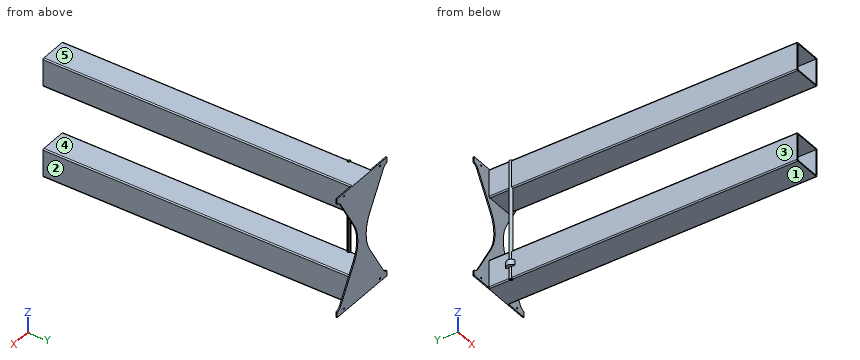
from build123d import *
from build123d.topology import SkipClean

# Parameters (mm, degrees)
SKETCH1_R           = 1.5875
BOSS_EXTRUDE1_DEPTH = 2.54
SKETCH2_W           = 63.5
SKETCH2_H           = 63.5
BOSS_EXTRUDE2_DEPTH = 685.8
SHELL1_START        = -688.34
SHELL1_OUTLINE_W    = 58.42
SHELL1_OUTLINE_H    = 58.42
SHELL1_DEPTH        = 685.8
FILLET1_R           = 2.54
FILLET2_R           = 2.54
CUT_EXTRUDE1_DEPTH  = 267.97
BOSS_EXTRUDE4_DEPTH = 27.94
BOSS_EXTRUDE5_DEPTH = 10.16
BOSS_EXTRUDE6_START = -0.762
BOSS_EXTRUDE6_DEPTH = 0.762
BOSS_EXTRUDE7_DEPTH = 0.762
BOSS_EXTRUDE8_DEPTH = 229.108
SKETCH12_W          = 2.54
SKETCH12_H          = 18.920978
CUT_EXTRUDE2_DEPTH  = 10.16


# Read off the part's stored shape, not the designer's step: Shell1
with BuildPart() as part:
    # Sketch1 → Boss-Extrude1 (new body)
    with BuildSketch(Plane(origin=(0, 0, 0), x_dir=(1, 0, 0), z_dir=(0, 1, 0))):
        with BuildLine():
            Line((-79.375, -133.985), (79.375, -133.985))
            Line((79.375, -133.985), (79.375, -123.618732))
            ThreePointArc((79.375, -123.618732), (78.770533, -121.973949), (77.244833, -121.112014))
            ThreePointArc((77.244833, -121.112014), (71.931312, -118.986411), (68.016546, -114.811929))
            Line((68.016546, -114.811929), (24.542449, -41.427653))
            ThreePointArc((24.542449, -41.427653), (13.192327, 0), (24.542449, 41.427653))
            Line((24.542449, 41.427653), (68.016546, 114.811929))
            ThreePointArc((68.016546, 114.811929), (71.931312, 118.986411), (77.244833, 121.112014))
            ThreePointArc((77.244833, 121.112014), (78.770533, 121.973949), (79.375, 123.618732))
            Line((79.375, 123.618732), (79.375, 133.985))
            Line((79.375, 133.985), (-79.375, 133.985))
            Line((-79.375, 133.985), (-79.375, 123.618732))
            ThreePointArc((-79.375, 123.618732), (-78.770533, 121.973949), (-77.244833, 121.112014))
            ThreePointArc((-77.244833, 121.112014), (-71.931312, 118.986411), (-68.016546, 114.811929))
            Line((-68.016546, 114.811929), (-24.542449, 41.427653))
            ThreePointArc((-24.542449, 41.427653), (-13.192327, 0), (-24.542449, -41.427653))
            Line((-24.542449, -41.427653), (-68.016546, -114.811929))
            ThreePointArc((-68.016546, -114.811929), (-71.931312, -118.986411), (-77.244833, -121.112014))
            ThreePointArc((-77.244833, -121.112014), (-78.770533, -121.973949), (-79.375, -123.618732))
            Line((-79.375, -123.618732), (-79.375, -133.985))
        make_face()
        with Locations(Location((-57.15, 127, 0), (0, 0, 270))):
            Circle(SKETCH1_R, mode=Mode.SUBTRACT)
        with Locations(Location((57.15, 127, 0), (0, 0, 270))):
            Circle(SKETCH1_R, mode=Mode.SUBTRACT)
        with Locations(Location((57.15, -127, 0), (0, 0, 90))):
            Circle(SKETCH1_R, mode=Mode.SUBTRACT)
        with Locations(Location((-57.15, -127, 0), (0, 0, 90))):
            Circle(SKETCH1_R, mode=Mode.SUBTRACT)
    extrude(amount=-BOSS_EXTRUDE1_DEPTH)

    # Sketch2 → Boss-Extrude2 (add)
    with BuildSketch(Plane.XZ.offset(2.54)):
        with Locations((0, -102.235)):
            Rectangle(SKETCH2_W, SKETCH2_H)
        with Locations((0, 102.235)):
            Rectangle(SKETCH2_W, SKETCH2_H)
    extrude(amount=BOSS_EXTRUDE2_DEPTH)

    # Shell1 outline → Shell1 (cut)
    with BuildSketch(Plane(origin=(0, 0, 0), x_dir=(1, 0, 0), z_dir=(0, 1, 0)).offset(SHELL1_START)):
        with Locations((0, 102.235)):
            Rectangle(SHELL1_OUTLINE_W, SHELL1_OUTLINE_H)
        with Locations((0, -102.235)):
            Rectangle(SHELL1_OUTLINE_W, SHELL1_OUTLINE_H)
    extrude(amount=SHELL1_DEPTH, mode=Mode.SUBTRACT)

    # Fillet1
    fillet1_edges = [part.edges().sort_by_distance(p)[0] for p in [
        (31.75, -345.44, 70.485),
        (31.75, -345.44, 133.985),
        (-31.75, -345.44, 133.985),
        (-31.75, -345.44, 70.485),
    ]]
    fillet(fillet1_edges, radius=FILLET1_R)

    # Fillet2
    fillet2_edges = [part.edges().sort_by_distance(p)[0] for p in [
        (-31.75, -345.44, -70.485),
        (-31.75, -345.44, -133.985),
        (31.75, -345.44, -133.985),
        (31.75, -345.44, -70.485),
    ]]
    fillet(fillet2_edges, radius=FILLET2_R)

    # Sketch4 → Cut-Extrude1 (cut)
    with BuildSketch(Plane(origin=(0, 0, -133.985), x_dir=(-1, 0, 0), z_dir=(0, 0, -1))):
        with BuildLine():
            ThreePointArc((29.21, -53.213), (31.455064, -52.283064), (32.385, -50.038))
            ThreePointArc((32.385, -50.038), (31.455064, -47.792936), (29.21, -46.863))
            Line((29.21, -46.863), (29.21, -53.213))
        make_face()
        with BuildLine():
            Line((29.21, -53.213), (29.21, -46.863))
            ThreePointArc((29.21, -46.863), (26.035, -50.038), (29.21, -53.213))
        make_face()
    extrude(amount=-CUT_EXTRUDE1_DEPTH, mode=Mode.SUBTRACT)

    # Sketch6 → Boss-Extrude4 (add)
    with BuildSketch(Plane(origin=(0, 0, -133.985), x_dir=(-1, 0, 0), z_dir=(0, 0, -1))):
        with BuildLine():
            Line((29.21, -46.863), (29.21, -46.228))
            ThreePointArc((29.21, -46.228), (33.02, -50.038), (29.21, -53.848))
            Line((29.21, -53.848), (29.21, -53.213))
            ThreePointArc((29.21, -53.213), (32.385, -50.038), (29.21, -46.863))
        make_face()
    extrude(amount=-BOSS_EXTRUDE4_DEPTH)

    # Sketch7 → Boss-Extrude5 (add)
    with BuildSketch(Plane.XY.offset(-106.045)):
        with BuildLine():
            ThreePointArc((-31.75, -40.069511), (-39.497, -50.038), (-31.75, -60.006489))
            Line((-31.75, -60.006489), (-31.75, -59.218089))
            ThreePointArc((-31.75, -59.218089), (-38.735, -50.038), (-31.75, -40.857911))
            Line((-31.75, -40.857911), (-31.75, -40.069511))
        make_face()
    extrude(amount=BOSS_EXTRUDE5_DEPTH)

    # Sketch7<2> → Boss-Extrude6 (add)
    with BuildSketch(Plane.XY.offset(-106.045).offset(BOSS_EXTRUDE6_START)):
        with BuildLine():
            ThreePointArc((-31.75, -40.069511), (-39.497, -50.038), (-31.75, -60.006489))
            Line((-31.75, -60.006489), (-31.75, -59.218089))
            ThreePointArc((-31.75, -59.218089), (-38.735, -50.038), (-31.75, -40.857911))
            Line((-31.75, -40.857911), (-31.75, -40.069511))
        make_face()
        with BuildLine():
            ThreePointArc((-31.75, -40.857911), (-38.735, -50.038), (-31.75, -59.218089))
            Line((-31.75, -59.218089), (-31.75, -52.877806))
            ThreePointArc((-31.75, -52.877806), (-33.02, -50.038), (-31.75, -47.198194))
            Line((-31.75, -47.198194), (-31.75, -40.857911))
        make_face()
    extrude(amount=BOSS_EXTRUDE6_DEPTH)

    # Sketch8 → Boss-Extrude7 (add)
    with SkipClean():  # the faces are left unmerged after this step: merging them gives an invalid solid
        with BuildSketch(Plane.XY.offset(-95.885)):
            with BuildLine():
                Line((-31.75, -40.069511), (-31.75, -48.133))
                ThreePointArc((-31.75, -48.133), (-32.385, -50.038), (-31.75, -51.943))
                Line((-31.75, -51.943), (-31.75, -60.006489))
                ThreePointArc((-31.75, -60.006489), (-39.497, -50.038), (-31.75, -40.069511))
            make_face()
        extrude(amount=BOSS_EXTRUDE7_DEPTH)

    # Sketch9 → Boss-Extrude8 (add)
    with SkipClean():  # the faces are left unmerged after this step: merging them gives an invalid solid
        with BuildSketch(Plane.XY.offset(-95.123)):
            with BuildLine():
                Line((-29.21, -46.228), (-29.21, -46.863))
                ThreePointArc((-29.21, -46.863), (-30.629903, -47.198194), (-31.75, -48.133))
                ThreePointArc((-31.75, -48.133), (-32.385, -50.038), (-31.75, -51.943))
                ThreePointArc((-31.75, -51.943), (-30.629903, -52.877806), (-29.21, -53.213))
                Line((-29.21, -53.213), (-29.21, -53.848))
                ThreePointArc((-29.21, -53.848), (-33.02, -50.038), (-29.21, -46.228))
            make_face()
        extrude(amount=BOSS_EXTRUDE8_DEPTH)

    # Sketch12 → Cut-Extrude2 (cut)
    with BuildSketch(Plane(origin=(0, 0, -95.885), x_dir=(-1, 0, 0), z_dir=(0, 0, -1))):
        with Locations((30.48, -50.038)):
            Rectangle(SKETCH12_W, SKETCH12_H)
    extrude(amount=CUT_EXTRUDE2_DEPTH, mode=Mode.SUBTRACT)


solid = part.part
Check sheet for the modelled part. Datum: model origin and axes. Units: mm. Face numbers are marked on the shaded views. A direction names the side the tool comes from. Round coordinates to 2 decimals unless told otherwise and drop trailing zeros. Write each loop counter-clockwise with the first axis right and the second up, starting at its lowest first coordinate (ties: lowest second). Pieces come first, ordered by that corner, then holes. Notation, with made-up numbers: (77.5, -13) -> (84.5, -13) arc R19 ccw to (84.5, 6) -> close; hole circle Ø9 at (24.5, 66.5). An arc over 180 degrees is marked (long way). Answer as CSV lines item,"result". Start each with the question number.
1) Section check B-B on z = -15.5. Enter the section's corners in (x, y) (3 decimals), and give its area (3 significant figures).
2) Section check A-A on y = -162. Enter the section's corners in (x, z) (3 decimals).
3) Section check C-C on x = -49. Enter the section's corners in (y, z) (3 decimals).
4) Section check D-D on x = -3. Enter the section's corners in (y, z) (3 decimals).
5) Material ranges on line 1 (X direction, y = -1, z = 127) (1 decimal); line 2 (Z direction, x = -4.5, y = -624.5) (3 decimals); line 3 (X direction, y = -635, z = 77), recorded low to high. Write a range as from..to.
6) Tool access check on the marked faces 1 and 2. Record the directions out of +Z, -Z, +X, -X, +Y, -Y that give a thin tool (end or side, any length) a straight path to the whole face; none if there is none.
7) Go/stop test with flat-tipped pins: P1, Ø10, axis at y = -291.5, z = -96.5, coming from the +X side; P2, Ø2.5, axis at x = -37.5, y = -49, coming from the +Z side; P3, Ø8.5, axis at x = -34, y = -49, coming from the -Z side (3 decimals); P4, Ø12, axis at x = -53.5, z = 85.5, coming from the -Y side. Record where each tip stops, or that it passes through.
8) Release check for a two-part mould opening along Z. For the marked faces 3, 4 and 5 record: pulls with the +Z half, pulls with the -Z half, needs draft (parallel to the pull), parting line crosses it, or undercut.
Found:
1,outline,"(-31.75, -51.943) arc R3.175 cw to (-31.75, -48.133) arc R3.175 cw to (-29.21, -46.863) -> (-29.21, -46.228) arc R3.81 ccw to (-29.21, -53.848) -> (-29.21, -53.213) arc R3.175 cw to start; (-14.684, -2.54) -> (14.684, -2.54) -> (14.684, 0) -> (-14.684, 0) -> close"
1,area,"81.6 mm^2"
2,outline,"(-31.75, -131.445) arc R2.54 ccw to (-29.21, -133.985) -> (29.21, -133.985) arc R2.54 ccw to (31.75, -131.445) -> (31.75, -73.025) arc R2.54 ccw to (29.21, -70.485) -> (-29.21, -70.485) arc R2.54 ccw to (-31.75, -73.025) -> close; (-31.75, 73.025) arc R2.54 ccw to (-29.21, 70.485) -> (29.21, 70.485) arc R2.54 ccw to (31.75, 73.025) -> (31.75, 131.445) arc R2.54 ccw to (29.21, 133.985) -> (-29.21, 133.985) arc R2.54 ccw to (-31.75, 131.445) -> close; hole (-29.21, -131.445) -> (29.21, -131.445) -> (29.21, -73.025) -> (-29.21, -73.025) -> close; hole (-29.21, 73.025) -> (29.21, 73.025) -> (29.21, 131.445) -> (-29.21, 131.445) -> close"
3,outline,"(-2.54, -133.985) -> (0, -133.985) -> (0, -82.712) -> (-2.54, -82.712) -> close; (-2.54, 82.712) -> (0, 82.712) -> (0, 133.985) -> (-2.54, 133.985) -> close"
4,outline,"(-688.34, -133.985) -> (0, -133.985) -> (0, 133.985) -> (-688.34, 133.985) -> (-688.34, 131.445) -> (-2.54, 131.445) -> (-2.54, 73.025) -> (-688.34, 73.025) -> (-688.34, 70.485) -> (-2.54, 70.485) -> (-2.54, -70.485) -> (-688.34, -70.485) -> (-688.34, -73.025) -> (-2.54, -73.025) -> (-2.54, -131.445) -> (-688.34, -131.445) -> close"
5,line 1,"x = -79.4..-58.7, -55.6..55.6, 58.7..79.4"
5,line 2,"z = -133.985..-131.445, -73.025..-70.485, 70.485..73.025, 131.445..133.985"
5,line 3,"x = -31.75..-29.21, 29.21..31.75"
6,face 1,"-Z, +X, -X, +Y, -Y"
6,face 2,"+Z, -Z, +X, -Y"
7,P1,"stops at x = 31.75"
7,P2,"stops at z = -95.12"
7,P3,"stops at z = -133.985"
7,P4,"stops at y = -2.54"
8,face 3,"needs draft"
8,face 4,"undercut"
8,face 5,"pulls with the +Z half"
